Read the model definition and answer for the solid it produces. Units are mm, in the model's axes. A direction names the side the tool comes from. Give positions to 0.01 mm unless a question says otherwise; leave off trailing zeros. Loops run counter-clockwise (first coordinate to the right, second up) from the corner with the lowest first, then second, coordinate; pieces in that order, holes last. Notation, with made-up numbers: (-13, 78) - (-8, 78) arc R21 ccw to (-8, 114) - close; hole circle Ø11 at (11, -28). An arc over 180 degrees is marked (long way). Write item = value, one per line.
```python
from build123d import *

# Parameters (mm, degrees)
SKETCH_R      = 4
SKETCH_R_2    = 2.5
PAD_DEPTH     = 4
SKETCH001_R   = 12
SKETCH001_R_2 = 4
PAD001_DEPTH  = 5
SKETCH002_R   = 6
SKETCH002_R_2 = 4
PAD002_DEPTH  = 4


with BuildPart() as part:
    # Sketch → Pad (new body)
    with BuildSketch(Plane.XZ):
        with BuildLine():
            ThreePointArc((5.655405, 12.258319), (0, 13.5), (-5.655405, 12.258319))
            Line((-20.908784, 5.221136), (-5.655405, 12.258319))
            ThreePointArc((-20.908784, 5.221136), (-24.25, 0), (-20.908784, -5.221136))
            Line((-20.908784, -5.221136), (-5.655405, -12.258319))
            ThreePointArc((-5.655405, -12.258319), (0, -13.5), (5.655405, -12.258319))
            Line((5.655405, -12.258319), (20.908784, -5.221136))
            ThreePointArc((20.908784, -5.221136), (24.25, 0), (20.908784, 5.221136))
            Line((5.655405, 12.258319), (20.908784, 5.221136))
        make_face()
        Circle(SKETCH_R, mode=Mode.SUBTRACT)
        with Locations((18.5, 0)):
            Circle(SKETCH_R_2, mode=Mode.SUBTRACT)
        with Locations((-18.5, 0)):
            Circle(SKETCH_R_2, mode=Mode.SUBTRACT)
    extrude(amount=PAD_DEPTH)

    # Sketch001 (on Face13 of Pad) → Pad001 (join)
    with BuildSketch(Plane.XZ.offset(4)):
        Circle(SKETCH001_R)
        Circle(SKETCH001_R_2, mode=Mode.SUBTRACT)
    extrude(amount=PAD001_DEPTH)

    # Sketch002 (on Face16 of Pad001) → Pad002 (join)
    with BuildSketch(Plane.XZ.offset(9)):
        Circle(SKETCH002_R)
        Circle(SKETCH002_R_2, mode=Mode.SUBTRACT)
    extrude(amount=PAD002_DEPTH)


solid = part.part
```
1) A tool of negligible diameter and unlimited length cuts with its end or side. For faces 1 (the face through (5, 0, 0)), 2 (the face through (7, -4, 10)), from which of +Z, -Z, +X, -X, +Y, -Y can it reach the whole face along a straight path? Write none if from no direction.
Output:
face_1 = +Z, -Z, +X, -X, +Y
face_2 = -Y
2) The mould has two halves that part along X. Classify faces 3 (the face through (16, -2, 0)), 4 (the face through (-6, -9, -2)), 5 (the face through (-0.1, -2, -13.5)): pulls with the +X half, pulls with the -X half, needs draft (parallel to the pull), parting line crosses it, or undercut.
Output:
face_3 = undercut
face_4 = needs draft
face_5 = parting line crosses it
3) A cutting plane is placed at D-D on x = 9.5. Determine the outline of the cut face in (y, z), then the cut area to 3 significant figures.
Output:
outline = (-9, -7.33) - (-4, -7.33) - (-4, -10.48) - (0, -10.48) - (0, 10.48) - (-4, 10.48) - (-4, 7.33) - (-9, 7.33) - close
area = 157 mm²
4) Each of these flat-tipped pins is pushed along its axis until it touches: P1, Ø3, axis at x = 18.5, z = 0, coming from the +Y side; P2, Ø6, axis at x = 14, y = -6.5, coming from the -Z side; P3, Ø2, axis at x = -3.5, y = -2.5, coming from the +Z side; P4, Ø1.5, axis at y = -1.5, z = 2, coming from the +X side. Where does it stop, or does it pass through?
Output:
P1 = through
P2 = -9.17
P3 = 13.27
P4 = 24.11
5) A cutting plane is placed at B-B on x = 0. Determine the outline of the cut face in (y, z), then the cut area to 3 significant figures.
Output:
outline = (-13, -6) - (-9, -6) - (-9, -12) - (-4, -12) - (-4, -13.5) - (0, -13.5) - (0, -4) - (-13, -4) - close; (-13, 4) - (0, 4) - (0, 13.5) - (-4, 13.5) - (-4, 12) - (-9, 12) - (-9, 6) - (-13, 6) - close
area = 172 mm²
6) A cutting plane is placed at C-C on y = -3.25. Determine the outline of the cut face in (x, z).
Output:
outline = (-20.91, -5.22) - (-5.66, -12.26) arc R13.5 ccw to (5.66, -12.26) - (20.91, -5.22) arc R5.75 ccw to (20.91, 5.22) - (5.66, 12.26) arc R13.5 ccw to (-5.66, 12.26) - (-20.91, 5.22) arc R5.75 ccw to start; hole circle Ø5 at (-18.5, 0); hole circle Ø8 at (0, 0); hole circle Ø5 at (18.5, 0)
7) Find the intervals of material crossed by probe 1 along Z at (x, y) = (0, -3.5); probe 2 along Y at (x, z) = (-7.5, -3); probe 3 along Z at (x, y) = (0, -6.25), in increasing order.
Output:
probe_1 = -13.5 to -4, 4 to 13.5
probe_2 = -9 to 0
probe_3 = -12 to -4, 4 to 12
8) A cutting plane is placed at A-A on z = 0. Determine the outline of the cut face in (x, y), then the cut area to 3 significant figures.
Output:
outline = (-24.25, -4) - (-21, -4) - (-21, 0) - (-24.25, 0) - close; (-16, -4) - (-12, -4) - (-12, -9) - (-6, -9) - (-6, -13) - (-4, -13) - (-4, 0) - (-16, 0) - close; (4, -13) - (6, -13) - (6, -9) - (12, -9) - (12, -4) - (16, -4) - (16, 0) - (4, 0) - close; (21, -4) - (24.25, -4) - (24.25, 0) - (21, 0) - close
area = 218 mm²
